Model file for the job. Use its own axes, mm. A direction names the side the tool comes from. Coordinates: 2 decimals unless noted, no trailing zeros. Write each loop counter-clockwise with the first axis right and the second up, starting at its lowest first coordinate (ties: lowest second). Pieces come first, ordered by that corner, then holes.
Q1. Pull direction X, two halves, no side cores. Call faces 1 (the flat face through (0, -7, -5.25)), 2 (the cylindrical face through (1.525, -0.632, 6.663)), 3 (the flat face through (14.516, 3, -4)): released by +X, released by -X, zero draft, split by the parting line, or undercut.
Q2. Drill centre lines: probe 1 along Y at (x, z) = (7.5, 0); probe 2 along Y at (x, z) = (0, -6.45); probe 3 along Z at (x, y) = (6.25, -0.5). Where is each one in solid material? Low to high.
Q3. Band-saw the part on A-A, the plane y = 0. Write the cut outline in (x, z).
Q4. Which spindle directions (+Z, -Z, +X, -X, +Y, -Y) get a long thin tool onto all of the face, cutting with end or side? Do faces 4 (the flat face through (0, 0, -6.05)), 5 (the cylindrical face through (0.135, 7.423, 4.859)), 6 (the flat face through (0, 7, -5.25)), 7 (the flat face through (0.1, 8.5, -0.404)), 8 (the cylindrical face through (-11.665, 1.938, 6.154)). Say none if no direction does.
Q5. Band-saw the part on B-B, the plane z = 0. Write the cut outline in (x, y).
Q6. Pin check, flat tips, straight feed: P1, Ø0.8, axis at x = -3, y = 7, coming from the +Z side; P2, Ø8, axis at x = 1.5, z = 5.5, coming from the +Y side; P3, Ø0.9, axis at x = 4.5, y = -8, coming from the -Z side; P4, Ø4, axis at x = 1.5, z = 2, coming from the +Y side. Stop position of each tip, or through.
from build123d import *

# Parameters (mm, degrees)
BOSS_EXTRUDE1_DEPTH      = 9.6774
BOSS_EXTRUDE1_DEPTH_BACK = 9.6774
SKETCH2_R                = 6.4516
BOSS_EXTRUDE2_DEPTH      = 4.8387
SKETCH3_R                = 6.4516
BOSS_EXTRUDE3_DEPTH      = 4.8387
SKETCH4_R                = 4.8387
CUT_EXTRUDE1_DEPTH       = 30.0322
FILLET1_R                = 0.80772
SKETCH5_R                = 1.651
CUT_EXTRUDE2_DEPTH       = 1.20904


with BuildPart() as part:
    # Sketch1 → Boss-Extrude1 (new body, two sides)
    with BuildSketch(Plane(origin=(0, 0, 0), x_dir=(0, 0, -1), z_dir=(1, 0, 0))) as boss_extrude1_sk:
        with BuildLine():
            Line((0.40386, 8.863023459), (0.40386, 8.054381252))
            ThreePointArc((0.40386, 8.054381252), (0.80874507, 8.023845192), (1.21158, 7.972968967))
            Line((1.21158, 7.972968967), (1.21158, 8.789104712))
            ThreePointArc((1.21158, 8.789104712), (1.617173927, 8.723590787), (2.0193, 8.639370072))
            Line((2.0193, 8.639370072), (2.0193, 7.807598079))
            ThreePointArc((2.0193, 7.807598079), (2.426507892, 7.690787977), (2.82702, 7.552755667))
            Line((2.82702, 7.552755667), (2.82702, 8.409770844))
            ThreePointArc((2.82702, 8.409770844), (3.234747336, 8.261519073), (3.63474, 8.093513011))
            Line((3.63474, 8.093513011), (3.63474, 7.19894613))
            ThreePointArc((3.63474, 7.19894613), (4.04538399, 6.976462472), (4.44246, 6.730580168))
            Line((4.44246, 6.730580168), (4.44246, 7.679898233))
            ThreePointArc((4.44246, 7.679898233), (4.853501008, 7.426965443), (5.25018, 7.152055487))
            Line((5.25018, 7.152055487), (5.25018, 6.121418971))
            ThreePointArc((5.25018, 6.121418971), (6.389316694, 4.920649595), (7.25932, 3.512610623))
            Line((7.25932, 3.512610623), (7.25932, -3.512610623))
            ThreePointArc((7.25932, -3.512610623), (6.389316694, -4.920649595), (5.25018, -6.121418971))
            Line((5.25018, -6.121418971), (5.25018, -7.152055487))
            ThreePointArc((5.25018, -7.152055487), (4.853501008, -7.426965443), (4.44246, -7.679898233))
            Line((4.44246, -7.679898233), (4.44246, -6.730580168))
            ThreePointArc((4.44246, -6.730580168), (4.04538399, -6.976462472), (3.63474, -7.19894613))
            Line((3.63474, -7.19894613), (3.63474, -8.093513011))
            ThreePointArc((3.63474, -8.093513011), (3.234747336, -8.261519073), (2.82702, -8.409770844))
            Line((2.82702, -8.409770844), (2.82702, -7.552755667))
            ThreePointArc((2.82702, -7.552755667), (2.426507892, -7.690787977), (2.0193, -7.807598079))
            Line((2.0193, -7.807598079), (2.0193, -8.639370072))
            ThreePointArc((2.0193, -8.639370072), (1.617173927, -8.723590787), (1.21158, -8.789104712))
            Line((1.21158, -8.789104712), (1.21158, -7.972968967))
            ThreePointArc((1.21158, -7.972968967), (0.80874507, -8.023845192), (0.40386, -8.054381252))
            Line((0.40386, -8.054381252), (0.40386, -8.863023459))
            ThreePointArc((0.40386, -8.863023459), (0, -8.87222), (-0.40386, -8.863023459))
            Line((-0.40386, -8.863023459), (-0.40386, -8.054381252))
            ThreePointArc((-0.40386, -8.054381252), (-0.80874507, -8.023845192), (-1.21158, -7.972968967))
            Line((-1.21158, -7.972968967), (-1.21158, -8.789104712))
            ThreePointArc((-1.21158, -8.789104712), (-1.617173927, -8.723590787), (-2.0193, -8.639370072))
            Line((-2.0193, -8.639370072), (-2.0193, -7.807598079))
            ThreePointArc((-2.0193, -7.807598079), (-2.426507892, -7.690787977), (-2.82702, -7.552755667))
            Line((-2.82702, -7.552755667), (-2.82702, -8.409770844))
            ThreePointArc((-2.82702, -8.409770844), (-3.234747336, -8.261519073), (-3.63474, -8.093513011))
            Line((-3.63474, -8.093513011), (-3.63474, -7.19894613))
            ThreePointArc((-3.63474, -7.19894613), (-4.04538399, -6.976462472), (-4.44246, -6.730580168))
            Line((-4.44246, -6.730580168), (-4.44246, -7.679898233))
            ThreePointArc((-4.44246, -7.679898233), (-4.853501008, -7.426965443), (-5.25018, -7.152055487))
            Line((-5.25018, -7.152055487), (-5.25018, -6.121418971))
            ThreePointArc((-5.25018, -6.121418971), (-6.389316694, -4.920649595), (-7.25932, -3.512610623))
            Line((-7.25932, -3.512610623), (-7.25932, 3.512610623))
            ThreePointArc((-7.25932, 3.512610623), (-6.389316694, 4.920649595), (-5.25018, 6.121418971))
            Line((-5.25018, 6.121418971), (-5.25018, 7.152055487))
            ThreePointArc((-5.25018, 7.152055487), (-4.853501008, 7.426965443), (-4.44246, 7.679898233))
            Line((-4.44246, 7.679898233), (-4.44246, 6.730580168))
            ThreePointArc((-4.44246, 6.730580168), (-4.04538399, 6.976462472), (-3.63474, 7.19894613))
            Line((-3.63474, 7.19894613), (-3.63474, 8.093513011))
            ThreePointArc((-3.63474, 8.093513011), (-3.234747336, 8.261519073), (-2.82702, 8.409770844))
            Line((-2.82702, 8.409770844), (-2.82702, 7.552755667))
            ThreePointArc((-2.82702, 7.552755667), (-2.426507892, 7.690787977), (-2.0193, 7.807598079))
            Line((-2.0193, 7.807598079), (-2.0193, 8.639370072))
            ThreePointArc((-2.0193, 8.639370072), (-1.617173927, 8.723590787), (-1.21158, 8.789104712))
            Line((-1.21158, 8.789104712), (-1.21158, 7.972968967))
            ThreePointArc((-1.21158, 7.972968967), (-0.80874507, 8.023845192), (-0.40386, 8.054381252))
            Line((-0.40386, 8.054381252), (-0.40386, 8.863023459))
            ThreePointArc((-0.40386, 8.863023459), (0, 8.87222), (0.40386, 8.863023459))
        make_face()
    extrude(amount=BOSS_EXTRUDE1_DEPTH)
    extrude(boss_extrude1_sk.sketch, amount=-BOSS_EXTRUDE1_DEPTH_BACK)

    # Sketch2 → Boss-Extrude2 (add)
    with BuildSketch(Plane(origin=(9.6774, 0, 0), x_dir=(0, 0, -1), z_dir=(1, 0, 0))):
        Circle(SKETCH2_R)
    extrude(amount=BOSS_EXTRUDE2_DEPTH)

    # Sketch3 → Boss-Extrude3 (add)
    with BuildSketch(Plane.ZY.offset(9.6774)):
        Circle(SKETCH3_R)
    extrude(amount=BOSS_EXTRUDE3_DEPTH)

    # Sketch4 → Cut-Extrude1 (cut, through all)
    with BuildSketch(Plane(origin=(14.5161, 0, 0), x_dir=(0, 0, -1), z_dir=(1, 0, 0))):
        Circle(SKETCH4_R)
    extrude(amount=-CUT_EXTRUDE1_DEPTH, mode=Mode.SUBTRACT)

    # Fillet1
    fillet1_edges = [part.edges().sort_by_distance(p)[0] for p in [
        (14.5161, 0, 6.4516),
        (-14.5161, 0, -6.4516),
    ]]
    fillet(fillet1_edges, radius=FILLET1_R)

    # Sketch5 → Cut-Extrude2 (cut)
    with BuildSketch(Plane.XY.offset(7.25932)):
        Circle(SKETCH5_R)
    cut_extrude2 = extrude(amount=-CUT_EXTRUDE2_DEPTH, mode=Mode.SUBTRACT)

    # Mirror1: Cut-Extrude2 across plane
    add(cut_extrude2.mirror(Plane.XY), mode=Mode.SUBTRACT)


solid = part.part
Answer sheet:
1. face 1: zero draft
1. face 2: undercut
1. face 3: released by +X
2. probe 1: y = -8.87 to -4.84, 4.84 to 8.87
2. probe 2: y = -4.84 to -1.65, 1.65 to 4.84
2. probe 3: z = -7.26 to -4.81, 4.81 to 7.26
3. outline: (-14.52, -5.64) arc R0.81 ccw to (-13.71, -6.45) - (-9.68, -6.45) - (-9.68, -7.26) - (-1.65, -7.26) - (-1.65, -6.05) - (1.65, -6.05) - (1.65, -7.26) - (9.68, -7.26) - (9.68, -6.45) - (13.71, -6.45) arc R0.81 ccw to (14.52, -5.64) - (14.52, -4.84) - (-14.52, -4.84) - close; (-14.52, 4.84) - (14.52, 4.84) - (14.52, 5.64) arc R0.81 ccw to (13.71, 6.45) - (9.68, 6.45) - (9.68, 7.26) - (1.65, 7.26) - (1.65, 6.05) - (-1.65, 6.05) - (-1.65, 7.26) - (-9.68, 7.26) - (-9.68, 6.45) - (-13.71, 6.45) arc R0.81 ccw to (-14.52, 5.64) - close
4. face 4: -Z
4. face 5: +Z, +X, -X, +Y
4. face 6: -Z, +X, -X, +Y
4. face 7: +X, -X, +Y
4. face 8: -X
5. outline: (-14.52, -5.64) arc R0.81 ccw to (-13.71, -6.45) - (-9.68, -6.45) - (-9.68, -8.87) - (9.68, -8.87) - (9.68, -6.45) - (13.71, -6.45) arc R0.81 ccw to (14.52, -5.64) - (14.52, -4.84) - (-14.52, -4.84) - close; (-14.52, 4.84) - (14.52, 4.84) - (14.52, 5.64) arc R0.81 ccw to (13.71, 6.45) - (9.68, 6.45) - (9.68, 8.87) - (-9.68, 8.87) - (-9.68, 6.45) - (-13.71, 6.45) arc R0.81 ccw to (-14.52, 5.64) - close
6. P1: stops at z = 5.25
6. P2: stops at y = 8.74
6. P3: stops at z = -4.66
6. P4: stops at y = 8.87
